Source: CAD feature listing. Evaluate the final solid. Frame: model axes, mm. Give positions to 0.01 mm unless a question says otherwise; leave off trailing zeros. Loops run counter-clockwise (first coordinate to the right, second up) from the corner with the lowest first, then second, coordinate; pieces in that order, holes last. Notation, with made-up numbers: M 47.5,-33 L 106.5,-33 A27 cw 106.5,1 Z; hole C -7,41.5 d8. An arc over 180 degrees is marked long. Answer in a Markdown table with one row per item.
Autodesk Inventor part; units mm, degrees
ref_plane "YZ Plane" through (0, 0, 0) normal (1, 0, 0) x (0, 1, 0)
ref_plane "XZ Plane" through (0, 0, 0) normal (0, 1, 0) x (-1, 0, 0)
ref_plane "XY Plane" through (0, 0, 0) normal (0, 0, 1) x (1, 0, 0)
sketch "Sketch1" plane through (0, 0, 0) normal (0, 0, 1) x (1, 0, 0)
  line L0 (-375, 30) -> (375, 30)
  line L1 (375, 30) -> (375, -30)
  line L2 (375, -30) -> (-375, -30)
  line L3 (-375, -30) -> (-375, 30)
  circle A0 centre (-240, 0) radius 5
  circle A1 centre (240, 0) radius 5
  point P0 (0, 0)
  dimension "d0" = 750
  dimension "d1" = 60
  dimension "d3" = 10
extrude "Extrusion1" add sketch "Sketch1" along normal blind 20
fillet "Fillet1" radius 30 1 edges at (0, 30, 20)
fillet "Fillet2" radius 10 4 edges at (-375, -14.1421, 20) (-375, 19.0362, 14.4949) (375, 19.0362, 14.4949) (375, -14.1421, 20)
properties part number "Topo_Aerofoil"
1) Section B-B, the plane x = 192.5. Return loops of the section in (y, z).
Reply:
| item | result |
|---|---|
| outline | M -30,0 L 30,0 A30 ccw 1.72,20 L -30,20 Z |
2) Material intervals for L1, parallel to X at y = 0, z = 3.75; L2, parallel to X at y = 0, z = 11.5; L3, parallel to Y at x = -240, z = 13.75, sorted ascending.
Reply:
| item | result |
|---|---|
| L1 | x = -375 to -245, -235 to 235, 245 to 375 |
| L2 | x = -374.89 to -245, -235 to 235, 245 to 374.89 |
| L3 | y = -30 to -5, 5 to 20.04 |
3) Pin query (flat end, axial travel): pin 1 Ø2 at (x, y) = (-40, -1.5) entering from -Z; pin 2 Ø3 at (y, z) = (23, 9.5) entering from -X; pin 3 Ø8 at (x, z) = (-103, 17.5) entering from +Y. Return the tip coordinate at first contact, or that it passes through.
Reply:
| item | result |
|---|---|
| pin 1 | stops at z = 0 |
| pin 2 | stops at x = -371.76 |
| pin 3 | stops at y = 20.36 |
4) Section A-A, the plane z = 13.25. Count the separate pieces of the cut face and the enclosed holes in it, then the cut area to 3 significant figures.
Reply:
| item | result |
|---|---|
| separate pieces | 1 |
| enclosed holes | 2 |
| area | 37,700 mm² |
